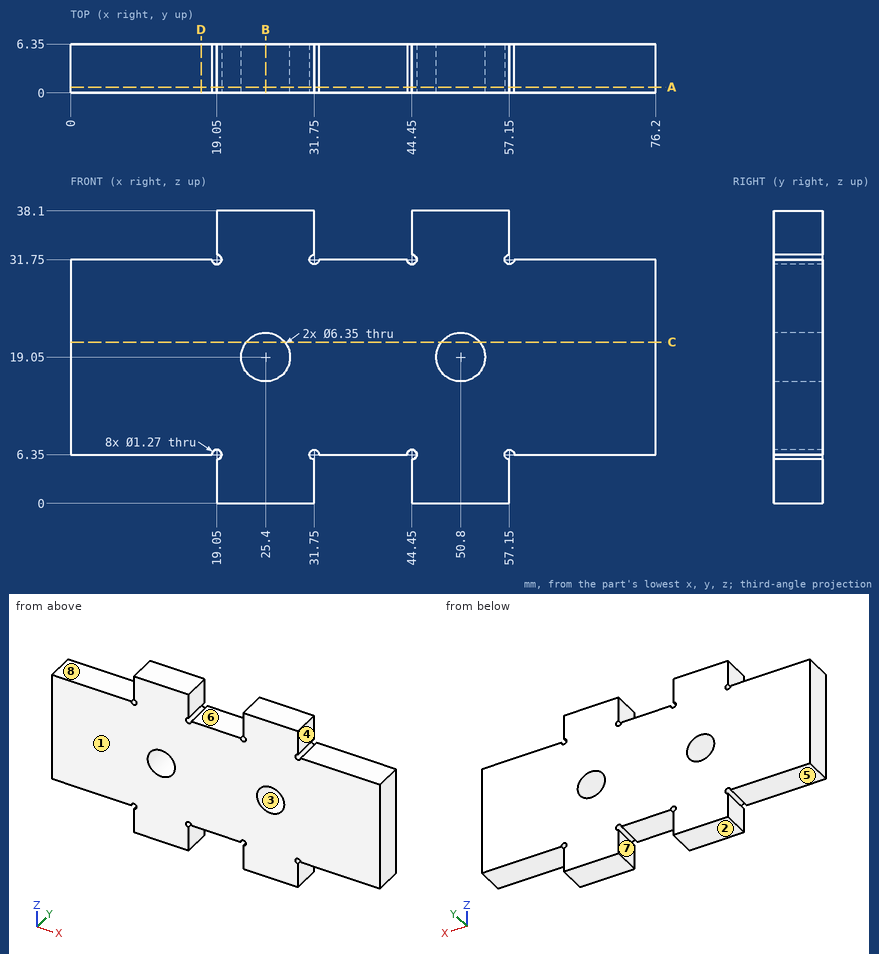
Could you check a few things on this drawing? It's one solid part, dimensions in mm from its lowest x, y, z. A direction names the side the tool comes from. Coordinates: 2 decimals unless noted, no trailing zeros. Order: outer loops, then holes, each group sorted by start corner. A loop starts at its lowest first (then second) coordinate and runs counter-clockwise, first axis right, second up. Notation, with made-up numbers: M 36,18.25 L 92,18.25 A5 cw 92,24.25 Z; hole C 0.25,75 d5. An arc over 180 degrees is marked long. Use a Markdown table: item, result. Add a question column.
Q1. Which directions (+Z, -Z, +X, -X, +Y, -Y) give clear straight access to the entire face, cutting with the end or side of a thin tool? Please do the marked faces 4, 5, 6, 7 and 8.
Q2. I want a section at C-C on z = 21. List the corners of the cut face in (x, y) for me, then the cut area to 3 significant figures.
Q3. I want a section at D-D on x = 17. List the corners of the cut face in (y, z) for me.
Q4. I want a section at A-A on y = 0.75. Give the number of separate pieces and of enclosed holes in the cut face, then the cut area to 3 significant figures.
Q5. If I drill on L1, parallel to X at y = 4, z = 19.05 (3 decimals); L2, parallel to X at y = 4.25, z = 18; L3, parallel to X at y = 4, z = 2, over which ranges is the centre line in solid material (lowest first)?
Q6. I'm going to push flat-ended pins straight in: pin 1 (1.7 mm diameter, centred on y = 3.5, z = 35, fed in from -X); pin 2 (3 mm diameter, centred on y = 2, z = 3.5, fed in from +X); pin 3 (1.5 mm diameter, centred on x = 19.05, z = 31.75, fed in from +Y); pin 4 (1.9 mm diameter, centred on x = 11.5, y = 4.5, fed in from -Z). Where does each tip first touch, or does it pass through?
Q7. I want a section at B-B on x = 25.4. List the corners of the cut face in (y, z) for me (3 decimals).
Q8. We'd pull the mould along Z, two halves only. Please class the marked faces 1, 2 and 3: pulls with the +Z half, pulls with the -Z half, needs draft (parallel to the pull), parting line crosses it, or undercut.
Checked values:
| question | item | result |
|---|---|---|
| 1 | face 4 | +Z, +X, +Y, -Y |
| 1 | face 5 | -Z, -X, +Y, -Y |
| 1 | face 6 | +Z, +Y, -Y |
| 1 | face 7 | -Z, +Y, -Y |
| 1 | face 8 | +Z, -X, +Y, -Y |
| 2 | outline | M 0,0 L 22.89,0 L 22.89,6.35 L 0,6.35 Z; M 27.91,0 L 48.29,0 L 48.29,6.35 L 27.91,6.35 Z; M 53.31,0 L 76.2,0 L 76.2,6.35 L 53.31,6.35 Z |
| 2 | area | 420 mm² |
| 3 | outline | M 0,6.35 L 6.35,6.35 L 6.35,31.75 L 0,31.75 Z |
| 4 | separate pieces | 1 |
| 4 | enclosed holes | 2 |
| 4 | area | 2,190 mm² |
| 5 | L1 | 0 to 22.225, 28.575 to 47.625, 53.975 to 76.2 |
| 5 | L2 | 0 to 22.4, 28.4 to 47.8, 53.8 to 76.2 |
| 5 | L3 | 19.05 to 31.75, 44.45 to 57.15 |
| 6 | pin 1 | x = 19.05 |
| 6 | pin 2 | x = 57.15 |
| 6 | pin 3 | y = 6.35 |
| 6 | pin 4 | z = 6.35 |
| 7 | outline | M 0,0 L 6.35,0 L 6.35,15.875 L 0,15.875 Z; M 0,22.225 L 6.35,22.225 L 6.35,38.1 L 0,38.1 Z |
| 8 | face 1 | needs draft |
| 8 | face 2 | pulls with the -Z half |
| 8 | face 3 | undercut |
